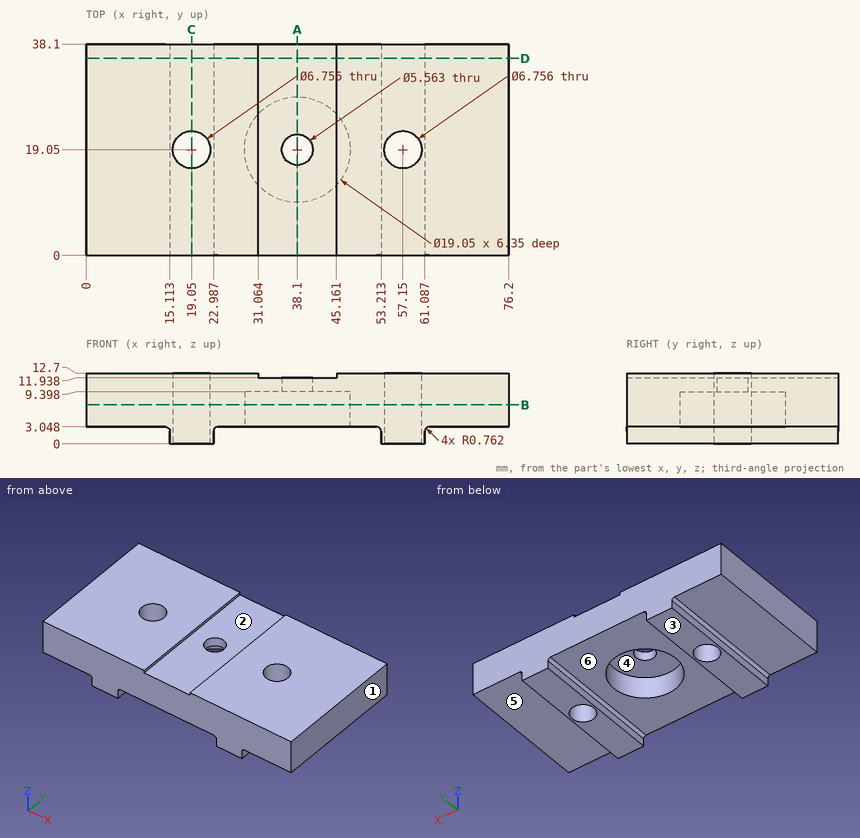
Verification items for this drawing (mm, ordinates from the low corner). A direction names the side the tool comes from. Coordinates: 2 decimals unless noted, no trailing zeros. Write each loop counter-clockwise with the first axis right and the second up, starting at its lowest first coordinate (ties: lowest second). Pieces come first, ordered by that corner, then holes. Notation, with made-up numbers: M 79,-34.75 L 104,-34.75 A17 cw 104,-3.75 Z; hole C 71.5,3.5 d3. An arc over 180 degrees is marked long. Answer as a JSON object with one key per item and string values. Group by question number.
(1) Release check for a two-part mould opening along X. For the marked faces 1, 2 and 3 record: +X half, -X half, draft (parallel to the pull), parting line (faces both ways), or undercut.
(2) Cross-section at D-D, the plane y = 35.5. Record the cut outline in (x, z) (1 decimal).
(3) Cross-section at A-A, the plane x = 38.1. Record the cut outline in (y, z) (1 decimal).
(4) Tool access check on the marked faces 4, 5 and 6. Record the directions out of +Z, -Z, +X, -X, +Y, -Y that give a thin tool (end or side, any length) a straight path to the whole face; none if there is none.
(5) Material ranges on line 1 (X direction, y = 19.05, z = 9.95); line 2 (X direction, y = 19.05, z = 7.75) (1 decimal); line 3 (Y direction, x = 19.05, z = 4.25), recorded low to high.
(6) Cross-section at C-C, the plane x = 19.05. Record the cut outline in (y, z).
(7) Cross-section at B-B, the plane z = 7. State how many separate pieces and enclosed holes the cut face has, and give its area (3 significant figures).
(8) Gauge pin test, flat ends, axial feed: pin 1 (5.5 mm diameter, centred on x = 35, y = 19, fed in from -Z); pin 2 (1.8 mm diameter, centred on y = 16.5, z = 1, fed in from +X); pin 3 (4 mm diameter, centred on x = 57.15, y = 19.05, fed in from -Z); pin 4 (1.1 mm diameter, centred on y = 12, z = 0.5, fed in from -X). Record the tip position at first contact, or that the pin passes through.
Reply:
{
 "1": {"face 1": "+X half", "face 2": "undercut", "face 3": "draft"},
 "2": {"outline": "M 0,3 L 14.4,3 A0.8 cw 15.1,2.3 L 15.1,0 L 23,0 L 23,2.3 A0.8 cw 23.7,3 L 52.5,3 A0.8 cw 53.2,2.3 L 53.2,0 L 61.1,0 L 61.1,2.3 A0.8 cw 61.8,3 L 76.2,3 L 76.2,12.7 L 45.2,12.7 L 45.2,11.9 L 31.1,11.9 L 31.1,12.7 L 0,12.7 Z"},
 "3": {"outline": "M 0,3 L 9.5,3 L 9.5,9.4 L 16.3,9.4 L 16.3,11.9 L 0,11.9 Z; M 21.8,9.4 L 28.6,9.4 L 28.6,3 L 38.1,3 L 38.1,11.9 L 21.8,11.9 Z"},
 "4": {"face 4": "-Z", "face 5": "-Z, +X, +Y, -Y", "face 6": "-Z, +Y, -Y"},
 "5": {"line 1": "0 to 15.67, 22.43 to 35.32, 40.88 to 53.77, 60.53 to 76.2", "line 2": "0 to 15.7, 22.4 to 28.6, 47.6 to 53.8, 60.5 to 76.2", "line 3": "0 to 15.67, 22.43 to 38.1"},
 "6": {"outline": "M 0,0 L 15.67,0 L 15.67,12.7 L 0,12.7 Z; M 22.43,0 L 38.1,0 L 38.1,12.7 L 22.43,12.7 Z"},
 "7": {"separate pieces": "1", "enclosed holes": "3", "area": "2,550 mm²"},
 "8": {"pin 1": "z = 9.4", "pin 2": "x = 61.09", "pin 3": "through", "pin 4": "x = 15.11"}
}
